Can you work these out from the model? Positions are in its coordinate system, mm. A direction names the side the tool comes from. Round coordinates to 2 decimals unless told otherwise and drop trailing zeros. Write each loop counter-clockwise with the first axis right and the second up, starting at its lowest first coordinate (ties: lowest second). Pieces come first, ordered by that corner, then holes. Notation, with made-up numbers: M 17,55.25 L 26,55.25 A15 cw 26,68.25 Z; hole C 48.5,86.25 d2. An arc over 180 degrees is marked long. Answer in a Markdown table with one row per item. Add a question column.
(1) Suppose I cut it at C-C, the plane z = 1.85. Count the separate pieces of the cut face and the enclosed holes in it, then the cut area to 3 significant figures.
(2) Suppose I cut it at B-B, the plane y = 32.75. Write out the boundary of the cut face in (x, z), then the cut area to 3 significant figures.
(3) If we mould it in two halves opening along X, with no side actions, what happens to faces 3 (the face through (-104.5, 14, 2)), 4 (the face through (32.038, 16.004, 2.348)), 5 (the face through (104.5, 14, 2))? For each: released by +X, released by -X, zero draft, split by the parting line, or undercut.
(4) Suppose I cut it at A-A, the plane x = 7.25. Write out the boundary of the cut face in (y, z).
(5) If I drill on probe 1 along Y at (x, z) = (-36, 3.4); probe 2 along X at (y, z) = (16.5, 0.55); probe 3 along X at (y, z) = (47, 2.2), over which ranges is the centre line in solid material (lowest first)?
(6) For faces 1 (the face through (70.57, 5.67, 2.35)), 2 (the face through (-92.381, 12.425, 2.348)), which set-ups out of +Z, -Z, +X, -X, +Y, -Y let a thin tool reach every point of the face, with its end or its side?
(7) Suppose I cut it at D-D, the plane x = -36. Write out the boundary of the cut face in (y, z).
(8) I'm going to push a flat-ended pin straight in: pin 1 (1.4 mm diameter, centred on x = 11, z = 2.5, fed in from -Y). Where does the tip first touch, or does it pass through?
from build123d import *

# Parameters (mm, degrees)
SKETCH_R   = 3
SKETCH_R_2 = 2.25
PAD_DEPTH  = 4.763


with BuildPart() as part:
    # Sketch → Pad (new body)
    with BuildSketch(Plane.XY):
        Polygon((-104.5, 0), (-104.5, 27.5), (-82.767832, 52.5), (82.767832, 52.5), (104.5, 27.5), (104.5, 0), (75.5, 0), (65.503203, 11.5), (-65.503203, 11.5), (-75.5, 0), align=None)
        with Locations((7.25, 39.75)):
            Circle(SKETCH_R, mode=Mode.SUBTRACT)
        with Locations((86, 32.75)):
            Circle(SKETCH_R, mode=Mode.SUBTRACT)
        with Locations((90, 14.25)):
            Circle(SKETCH_R, mode=Mode.SUBTRACT)
        with Locations((-90, 14.25)):
            Circle(SKETCH_R, mode=Mode.SUBTRACT)
        with Locations((-86, 32.75)):
            Circle(SKETCH_R, mode=Mode.SUBTRACT)
        with Locations((-36, 45.5)):
            Circle(SKETCH_R_2, mode=Mode.SUBTRACT)
        with Locations((-36, 18)):
            Circle(SKETCH_R_2, mode=Mode.SUBTRACT)
        with Locations((31, 18)):
            Circle(SKETCH_R_2, mode=Mode.SUBTRACT)
        with Locations((31, 45.5)):
            Circle(SKETCH_R_2, mode=Mode.SUBTRACT)
    extrude(amount=PAD_DEPTH)


solid = part.part
Calculated:
| question | item | result |
|---|---|---|
| 1 | separate pieces | 1 |
| 1 | enclosed holes | 9 |
| 1 | area | 8,600 mm² |
| 2 | outline | M -99.94,0 L -89,0 L -89,4.76 L -99.94,4.76 Z; M -83,0 L 83,0 L 83,4.76 L -83,4.76 Z; M 89,0 L 99.94,0 L 99.94,4.76 L 89,4.76 Z |
| 2 | area | 895 mm² |
| 3 | face 3 | released by -X |
| 3 | face 4 | undercut |
| 3 | face 5 | released by +X |
| 4 | outline | M 11.5,0 L 36.75,0 L 36.75,4.76 L 11.5,4.76 Z; M 42.75,0 L 52.5,0 L 52.5,4.76 L 42.75,4.76 Z |
| 5 | probe 1 | 11.5 to 15.75, 20.25 to 43.25, 47.75 to 52.5 |
| 5 | probe 2 | -104.5 to -91.98, -88.02 to -37.68, -34.32 to 29.32, 32.68 to 88.02, 91.98 to 104.5 |
| 5 | probe 3 | -87.55 to -37.68, -34.32 to 29.32, 32.68 to 87.55 |
| 6 | face 1 | +Z, -Z, -Y |
| 6 | face 2 | +Z, -Z |
| 7 | outline | M 11.5,0 L 15.75,0 L 15.75,4.76 L 11.5,4.76 Z; M 20.25,0 L 43.25,0 L 43.25,4.76 L 20.25,4.76 Z; M 47.75,0 L 52.5,0 L 52.5,4.76 L 47.75,4.76 Z |
| 8 | pin 1 | y = 11.5 |
